```python
from build123d import *

# Parameters (mm, degrees)
EXTRUDE_1_DEPTH          = 30
CUT_EXTRUDE_1_DEPTH      = 54.946640303
CUT_EXTRUDE_1_DEPTH_BACK = 54.946640303
SKETCH_2_W               = 42
SKETCH_2_H               = 12
CUT_EXTRUDE_4_REACH      = 55.947
SKETCH_3_R               = 1.5
SKETCH_5_R               = 1.475
CUT_EXTRUDE_5_DEPTH      = 5
CUT_EXTRUDE_7_DEPTH      = 2.4
FILLET_1_R               = 1
FILLET_5_R               = 0.5
FILLET_7_R               = 2


with BuildPart() as part:
    # 草圖1 → 填料-伸長1 (new, symmetric)
    with BuildSketch(Plane.XY):
        Polygon((-43, 0), (-43, 3), (-37.5, 3), (-37.5, 10), (-43.2, 10), (-43.2, 12), (41.8, 12), (41.8, 10), (37.5, 10), (37.5, 3), (43, 3), (43, 0), (35.5, 0), (35.5, 10), (-35.5, 10), (-35.5, 0), align=None)
    extrude(amount=EXTRUDE_1_DEPTH, both=True)

    # 草圖2 → 除料-伸長1 (cut, two sides: drawn at the far end of the back side and taken through both)
    with BuildSketch(Plane(origin=(0, 0, 0), x_dir=(0, 0, -1), z_dir=(1, 0, 0)).offset(-CUT_EXTRUDE_1_DEPTH_BACK)):
        Rectangle(SKETCH_2_W, SKETCH_2_H)
    extrude(amount=CUT_EXTRUDE_1_DEPTH + CUT_EXTRUDE_1_DEPTH_BACK, mode=Mode.SUBTRACT)

    # 草圖3 → 除料-伸長4 (cut, up to next)
    with BuildSketch(Plane(origin=(0, 0, 0), x_dir=(1, 0, 0), z_dir=(0, 1, 0)), mode=Mode.PRIVATE) as cut_extrude_4_sk1:
        with Locations(Location((-40, 25.5, 0), (0, 0, 90))):
            Circle(SKETCH_3_R)
    cut_extrude_4_tool1 = extrude(cut_extrude_4_sk1.sketch, amount=CUT_EXTRUDE_4_REACH, mode=Mode.PRIVATE) & part.part
    # 草圖3 → 除料-伸長4 (cut, up to next)
    with BuildSketch(Plane(origin=(0, 0, 0), x_dir=(1, 0, 0), z_dir=(0, 1, 0)), mode=Mode.PRIVATE) as cut_extrude_4_sk2:
        with Locations(Location((40, 25.5, 0), (0, 0, 90))):
            Circle(SKETCH_3_R)
    cut_extrude_4_tool2 = extrude(cut_extrude_4_sk2.sketch, amount=CUT_EXTRUDE_4_REACH, mode=Mode.PRIVATE) & part.part
    # 草圖3 → 除料-伸長4 (cut, up to next)
    with BuildSketch(Plane(origin=(0, 0, 0), x_dir=(1, 0, 0), z_dir=(0, 1, 0)), mode=Mode.PRIVATE) as cut_extrude_4_sk3:
        with Locations(Location((40, -25.5, 0), (0, 0, 90))):
            Circle(SKETCH_3_R)
    cut_extrude_4_tool3 = extrude(cut_extrude_4_sk3.sketch, amount=CUT_EXTRUDE_4_REACH, mode=Mode.PRIVATE) & part.part
    # 草圖3 → 除料-伸長4 (cut, up to next)
    with BuildSketch(Plane(origin=(0, 0, 0), x_dir=(1, 0, 0), z_dir=(0, 1, 0)), mode=Mode.PRIVATE) as cut_extrude_4_sk4:
        with Locations(Location((-40, -25.5, 0), (0, 0, 90))):
            Circle(SKETCH_3_R)
    cut_extrude_4_tool4 = extrude(cut_extrude_4_sk4.sketch, amount=CUT_EXTRUDE_4_REACH, mode=Mode.PRIVATE) & part.part
    add(cut_extrude_4_tool1.solids().sort_by_distance((-40, 0, -25.5))[0], mode=Mode.SUBTRACT)
    add(cut_extrude_4_tool2.solids().sort_by_distance((40, 0, -25.5))[0], mode=Mode.SUBTRACT)
    add(cut_extrude_4_tool3.solids().sort_by_distance((40, 0, 25.5))[0], mode=Mode.SUBTRACT)
    add(cut_extrude_4_tool4.solids().sort_by_distance((-40, 0, 25.5))[0], mode=Mode.SUBTRACT)

    # 草圖5 → 除料-伸長5 (cut)
    with BuildSketch(Plane(origin=(0, 12, 0), x_dir=(1, 0, 0), z_dir=(0, 1, 0))):
        with Locations(Location((-40.2, 24.5, 0), (0, 0, 270))):
            Circle(SKETCH_5_R)
        with Locations(Location((-40.2, -24.5, 0), (0, 0, 270))):
            Circle(SKETCH_5_R)
        with Locations(Location((17.8, 24.5, 0), (0, 0, 270))):
            Circle(SKETCH_5_R)
        with Locations(Location((17.8, -24.5, 0), (0, 0, 270))):
            Circle(SKETCH_5_R)
    extrude(amount=-CUT_EXTRUDE_5_DEPTH, mode=Mode.SUBTRACT)

    # 草圖16 → 除料-伸長7 (cut)
    with BuildSketch(Plane.XZ):
        Polygon((-40, 22.209103466), (-37.15, 23.854551733), (-37.15, 27.145448267), (-40, 28.790896534), (-42.85, 27.145448267), (-42.85, 23.854551733), align=None)
        Polygon((-42.85, -23.854551733), (-40, -22.209103466), (-37.15, -23.854551733), (-37.15, -27.145448267), (-40, -28.790896534), (-42.85, -27.145448267), align=None)
        Polygon((40, -22.209103466), (37.15, -23.854551733), (37.15, -27.145448267), (40, -28.790896534), (42.85, -27.145448267), (42.85, -23.854551733), align=None)
        Polygon((42.85, 23.854551733), (40, 22.209103466), (37.15, 23.854551733), (37.15, 27.145448267), (40, 28.790896534), (42.85, 27.145448267), align=None)
    extrude(amount=-CUT_EXTRUDE_7_DEPTH, mode=Mode.SUBTRACT)

    # 圓角1
    fillet_1_edges = [part.edges().sort_by_distance(p)[0] for p in [
        (-43, 1.5, -30),
        (-43.2, 11, -30),
        (41.8, 11, -30),
        (43, 1.5, -30),
        (43, 1.5, 30),
        (41.8, 11, 30),
        (-43, 1.5, 21),
        (-43, 1.5, -21),
        (-43.2, 11, 30),
        (43, 1.5, -21),
        (43, 1.5, 21),
        (-43, 1.5, 30),
    ]]
    fillet(fillet_1_edges, radius=FILLET_1_R)

    # 圓角5
    fillet_5_edges = [part.edges().sort_by_distance(p)[0] for p in [
        (-37.5, 3, 25.5),
        (37.5, 3, 25.5),
        (-37.5, 3, -25.5),
        (37.5, 3, -25.5),
    ]]
    fillet(fillet_5_edges, radius=FILLET_5_R)

    # 圓角7
    fillet_7_edges = [part.edges().sort_by_distance(p)[0] for p in [
        (35.5, 10, 0),
        (-35.5, 10, 0),
    ]]
    fillet(fillet_7_edges, radius=FILLET_7_R)


solid = part.part
```
For this review, take the finished solid that the model builds, in its own axes (mm). A direction names the side the tool comes from. Give positions to 0.01 mm unless a question says otherwise; leave off trailing zeros. Write each loop counter-clockwise with the first axis right and the second up, starting at its lowest first coordinate (ties: lowest second). Pieces come first, ordered by that corner, then holes. Notation, with made-up numbers: M -5.75,17.5 L 10.25,17.5 A23 cw 10.25,41.5 Z; hole C -34,-7 d6. An arc over 180 degrees is marked long. Answer as CSV lines item,"result".
1. Draft analysis for pull direction Y (two halves, no side actions). For faces 4 (the flat face through (42, 3, -25)), 5 (the flat face through (0, 10, 0)), 6 (the flat face through (-43.2, 11, 0)), state which applies: +Y half, -Y half, draft (parallel to the pull), parting line (faces both ways), or undercut.
Findings:
face 4,"undercut"
face 5,"-Y half"
face 6,"draft"
2. For pin 1 (5 mm diameter, centred on y = 4, z = -2.5, fed in from -X); pin 2 (5 mm diameter, centred on y = 8.5, z = -12.5, fed in from +X); pin 3 (3.5 mm diameter, centred on y = 1, z = 25.5, fed in from -X); pin 4 (1.5 mm diameter, centred on x = 9, y = 8.5, fed in from -Z), all flat-tipped, find the tip position at first contact; note any pin that passes through.
Findings:
pin 1,"stops at x = -37.5"
pin 2,"stops at x = 41.8"
pin 3,"stops at x = -43"
pin 4,"passes through"
3. For faces 1 (the flat face through (37.15, 1, -25)), 2 (the flat face through (-42, 3, -25)), 3 (the flat face through (36, 6, 0)), list the 3-axis set-ups (+Z, -Z, +X, -X, +Y, -Y) from which the entire face can be reached by the end or side of a thin tool; tool diameter is ignored.
Findings:
face 1,"-Y"
face 2,"+Z, -Z, -X"
face 3,"+X, -X, -Y"
4. Consider section A-A, the plane y = 1.5. Count the separate pieces of the cut face and the enclosed holes in it, then the cut area to 3 significant figures.
Findings:
separate pieces,"4"
enclosed holes,"4"
area,"156 mm2"
5. Wall thickness on line 1 (X direction, y = 2.7, z = -25.5); line 2 (X direction, y = 11.2, z = 24.5) (3 decimals); line 3 (X direction, y = 8.25, z = -15.5): over which ranges is each line inside the solid? List them lowest first.
Findings:
line 1,"x = -43 to -41.5, -38.5 to -35.5, 35.5 to 38.5, 41.5 to 43"
line 2,"x = -43.2 to -41.675, -38.725 to 16.325, 19.275 to 41.8"
line 3,"x = -37.5 to -35.48, 35.48 to 37.5"
6. Consider section B-B, the plane z = 10. Write out the cut boundary in (x, y), then the cut area to 3 significant figures.
Findings:
outline,"M -43.2,10 L -37.5,10 L -37.5,6 L -35.5,6 L -35.5,8 A2 cw -33.5,10 L 33.5,10 A2 cw 35.5,8 L 35.5,6 L 37.5,6 L 37.5,10 L 41.8,10 L 41.8,12 L -43.2,12 Z"
area,"188 mm2"
7. Consider section C-C, the plane x = -21. Write out the cut boundary in (y, z), then the cut area to 3 significant figures.
Findings:
outline,"M 10,-30 L 12,-30 L 12,30 L 10,30 Z"
area,"120 mm2"
